Model file for the job. Use its own axes, mm. Face numbers are marked on the shaded views. A direction names the side the tool comes from. Coordinates: 2 decimals unless noted, no trailing zeros. Write each loop counter-clockwise with the first axis right and the second up, starting at its lowest first coordinate (ties: lowest second). Pieces come first, ordered by that corner, then holes.
Q1. Band-saw the part on D-D, the plane z = -6.5. Write the cut outline in (x, y).
Q2. Which spindle directions (+Z, -Z, +X, -X, +Y, -Y) get a long thin tool onto all of the face, cutting with end or side? Do the marked faces 1, 2 and 3. Say none if no direction does.
Q3. Pull direction X, two halves, no side cores. Call the marked faces 4, 5 and 6: released by +X, released by -X, zero draft, split by the parting line, or undercut.
Q4. Pin check, flat tips, straight feed: P1, Ø4.5, axis at y = -7, z = -8, coming from the +X side; P2, Ø7, axis at x = -5.5, z = 1.5, coming from the +Y side; P3, Ø2.5, axis at y = -7, z = -8, coming from the +X side; P4, Ø8, axis at x = 11.5, y = -8, coming from the -Z side. Stop position of each tip, or through.
Q5. Drill centre lines: probe 1 along X at (y, z) = (-5.75, -9.75); probe 2 along Y at (x, z) = (-17.1, -8); probe 3 along Y at (x, z) = (11.5, 2). Where is each one in solid material? Low to high.
Q6. Band-saw the part on B-B, the plane y = -4.5. Write the cut outline in (x, z).
Q7. Band-saw the part on A-A, the plane x = -3.5. Write the cut outline in (y, z), plus the area to 3 significant figures.
Q8. Band-saw the part on C-C, the plane z = -2.25. Write the cut outline in (x, y), plus the area to 3 significant figures.
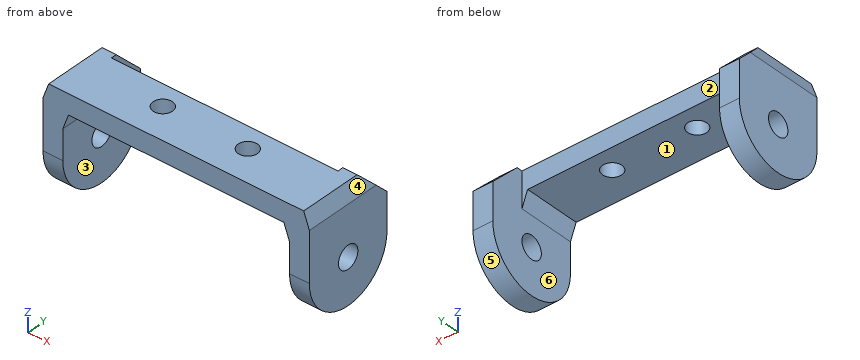
from build123d import *
from OCP.BRepFilletAPI import BRepFilletAPI_MakeChamfer

# Parameters (mm, degrees)
SKETCH_1_W          = 47
SKETCH_1_H          = 16
EXTRUDE_1_DEPTH     = 3.5
SKETCH_2_R          = 2
EXTRUDE_2_DEPTH     = 3.5
SKETCH_3_R          = 1.7
CUT_EXTRUDE_1_DEPTH = 10
SKETCH_4_W          = 40
SKETCH_4_H          = 6
CUT_EXTRUDE_2_DEPTH = 10
CHAMFER_4_SIZE      = 1
CHAMFER_4_SIZE2     = 2.747477419
CHAMFER1_SIZE       = 5


with BuildPart() as part:
    # 草图1 → 凸台-拉伸1 (new body)
    with BuildSketch(Plane.XY):
        with Locations((4, -7)):
            Rectangle(SKETCH_1_W, SKETCH_1_H)
    extrude(amount=EXTRUDE_1_DEPTH)

    # 草图2 → 凸台-拉伸2 (add)
    with BuildSketch(Plane(origin=(27.5, 0, 0), x_dir=(0, 0, -1), z_dir=(1, 0, 0))):
        with BuildLine():
            Line((0, 1), (0, -15))
            Line((0, -15), (8, -15))
            ThreePointArc((8, -15), (16, -7), (8, 1))
            Line((8, 1), (0, 1))
        make_face()
        with Locations((8, -7)):
            Circle(SKETCH_2_R, mode=Mode.SUBTRACT)
    extrude_2 = extrude(amount=-EXTRUDE_2_DEPTH)

    # 镜向1: 凸台-拉伸2 across plane
    add(extrude_2.mirror(Plane.ZY.offset(-4)))

    # 草图3 → 切除-拉伸1 (cut)
    with BuildSketch(Plane.XY.offset(3.5)):
        with Locations((11.5, -9)):
            Circle(SKETCH_3_R)
        with Locations((-3.5, -9)):
            Circle(SKETCH_3_R)
    extrude(amount=-CUT_EXTRUDE_1_DEPTH, mode=Mode.SUBTRACT)

    # 草图4 → 切除-拉伸2 (cut)
    with BuildSketch(Plane.XY.offset(3.5)):
        with Locations((4, -2)):
            Rectangle(SKETCH_4_W, SKETCH_4_H)
    extrude(amount=-CUT_EXTRUDE_2_DEPTH, mode=Mode.SUBTRACT)

    # 倒角4: one chamfer whose edges measure the first distance from different faces: ONE call of the kernel's chamfer builder (chamfer() names one face for all edges)
    chamfer_4_edges_1 = [part.edges().sort_by_distance(p)[0] for p in [
        (27.5, -7, 3.5),
        (-19.5, -7, 3.5),
    ]]
    chamfer_4_side_1 = [part.faces().sort_by_distance(p)[0] for p in [
        (4, -9.356389583, 3.5),
    ]]
    chamfer_4_edges_2 = [part.edges().sort_by_distance(p)[0] for p in [
        (-16, -10, 0),
        (24, -10, 0),
    ]]
    chamfer_4_side_2 = [part.faces().sort_by_distance(p)[0] for p in [
        (4, -10.047554813, 0),
    ]]
    chamfer_4 = BRepFilletAPI_MakeChamfer(part.part.solid().wrapped)
    for e in chamfer_4_edges_1:
        chamfer_4.Add(CHAMFER_4_SIZE, CHAMFER_4_SIZE2, e.wrapped, chamfer_4_side_1[0].wrapped)  # the first distance lies on this face
    for e in chamfer_4_edges_2:
        chamfer_4.Add(CHAMFER_4_SIZE, CHAMFER_4_SIZE2, e.wrapped, chamfer_4_side_2[0].wrapped)  # the first distance lies on this face
    add(Compound.cast(chamfer_4.Shape()), mode=Mode.REPLACE)

    # Chamfer1
    chamfer1_edges = [part.edges().sort_by_distance(p)[0] for p in [
        (-17.25, 1, 3.5),
        (25.25, 1, 3.5),
    ]]
    chamfer(chamfer1_edges, length=CHAMFER1_SIZE)


solid = part.part
Answer sheet:
1. outline: (-19.5, -15) - (-16, -15) - (-16, -8.32) - (-19.5, -8.32) - close; (-19.5, -5.68) - (-16, -5.68) - (-16, 1) - (-19.5, 1) - close; (24, -15) - (27.5, -15) - (27.5, -8.32) - (24, -8.32) - close; (24, -5.68) - (27.5, -5.68) - (27.5, 1) - (24, 1) - close
2. face 1: -Z, +Y, -Y
2. face 2: +Z, -Z, +Y
2. face 3: -Z, +Y
3. face 4: released by +X
3. face 5: zero draft
3. face 6: undercut
4. P1: stops at x = 27.5
4. P2: stops at y = -5
4. P3: passes through
4. P4: stops at z = 0
5. probe 1: x = -19.5 to -16, 24 to 27.5
5. probe 2: y = -15 to -9, -5 to 1
5. probe 3: y = -15 to -10.7, -7.3 to -5
6. outline: (-19.5, -15.6) - (-16, -15.6) - (-16, 3.5) - (-18.5, 3.5) - (-19.5, 0.75) - close; (24, -15.6) - (27.5, -15.6) - (27.5, 0.75) - (26.5, 3.5) - (24, 3.5) - close
7. outline: (-15, 0) - (-10.7, 0) - (-10.7, 3.5) - (-15, 3.5) - close; (-7.3, 0) - (-5, 0) - (-5, 3.5) - (-7.3, 3.5) - close
7. area: 23.1 mm2
8. outline: (-19.5, -15) - (-15.82, -15) - (-15.82, -5) - (-16, -5) - (-16, 1) - (-19.5, 1) - close; (23.82, -15) - (27.5, -15) - (27.5, 1) - (24, 1) - (24, -5) - (23.82, -5) - close
8. area: 116 mm2
